Autodesk Inventor part; units mm, degrees
ref_plane "YZ Plane" through (0, 0, 0) normal (1, 0, 0) x (0, 1, 0)
ref_plane "XZ Plane" through (0, 0, 0) normal (0, 1, 0) x (-1, 0, 0)
ref_plane "XY Plane" through (0, 0, 0) normal (0, 0, 1) x (1, 0, 0)
sketch "Sketch1" plane through (0, 0, 0) normal (0, 1, 0) x (-1, 0, 0)
  circle A0 centre (0, 35) radius 7.5
  circle A1 centre (0, -35) radius 7.5
  circle A2 centre (0, 0) radius 6
  dimension "d0" = 15
  dimension "d1" = 35
  dimension "d2" = 15
  dimension "d3" = 35
  dimension "d4" = 12
sketch "Sketch2" plane through (0, 0, 0) normal (0, 1, 0) x (-1, 0, 0)
  line L0 (12, 40) -> (12, -40)
  line L1 (12, -40) -> (5, -55)
  line L2 (12, 40) -> (5, 55)
  line L3 (0, 53.0774) -> (0, -54.9051) construction
  line L4 (-12, 40) -> (-12, -40)
  line L5 (-12, -40) -> (-5, -55)
  line L6 (-12, 40) -> (-5, 55)
  arc A0 (5, 55) -> (-5, 55) centre (0, 52.6667) ccw
  arc A1 (-5, -55) -> (5, -55) centre (0, -52.6667) ccw
  point P0 (0, 0)
  dimension "d5" = 12
  dimension "d6" = 40
  dimension "d7" = 40
  dimension "d8" = 15
  dimension "d9" = 7
  dimension "d10" = 15
  dimension "d11" = 7
extrude "Extrusion1" add sketch "Sketch2" along normal blind 15
extrude "Extrusion2" cut sketch "Sketch1" along normal blind 10
sketch "Sketch3" plane through (0, 0, 0) normal (0, -1, 0) x (1, 0, 0)
  point P0 (0, 0)
  point P1 (0, -50)
  point P2 (0, 50)
  dimension "d16" = 50
  dimension "d17" = 50
hole "Hole1" at (0, 0, -50) at (0, 0, 50) direction (0, 1, 0) diameter 4 end through all counterbore diameter 5 counterbore depth 2
properties part number "Rahmen_Y_Halterung_v1"
Here's how the part is built. I have some questions about the finished solid (model axes, mm). A direction names the side the tool comes from. Give positions to 0.01 mm unless a question says otherwise; leave off trailing zeros. Loops run counter-clockwise (first coordinate to the right, second up) from the corner with the lowest first, then second, coordinate; pieces in that order, holes last. Notation, with made-up numbers: (25, -19.75) -> (51, -19.75) arc R10 cw to (51, -6.75) -> close; hole circle Ø6 at (-22, -30). An arc over 180 degrees is marked (long way). Use one line per item in the form item = value. Start each with the question number.
1) Imagine slicing it at B-B (z = -50). Please give me the cut outline in (x, y), then the cut area to 3 significant figures.
2) Which directions (+Z, -Z, +X, -X, +Y, -Y) give clear straight access to the entire face, cutting with the end or side of a thin tool? Please do faces 4 (the face through (-2, 2, 51)), 5 (the face through (12, 7, 1)).
3) Please list where these lines run through material, in increasing order: line 1 along Z through (x, y) = (1, 1.5); line 2 along Z through (x, y) = (2.25, 8.5).
4) Imagine slicing it at A-A (x = 0). Count the separate pieces of the cut face and the enclosed holes in it, then the cut area to 3 significant figures.
5) Imagine slicing it at D-D (z = 35). Please give me the cut outline in (x, y).
6) Thinking about a two-plate mould opening in X: for faces 1 (the face through (8.549, 7.395, -47.395)), 2 (the face through (0.766, 8.591, -51.847)), 3 (the face through (-8.549, 7.395, 47.395)), which applies, +X half, -X half, draft (parallel to the pull), parting line (faces both ways), or undercut?
7) Imagine slicing it at C-C (y = 3). Please give me the cut outline in (x, z).
8) For P1, Ø6, axis at x = 6, y = 4, coming from the -Z side; P2, Ø7.5, axis at x = 1.5, z = -37, coming from the -Y side; P3, Ø1.5, axis at x = 1, z = -49, coming from the -Y side, each with a flat end and sliding along its axis, tell me the tip position at first contact or that it passes through.
Check values:
q1.outline = (-7.33, 0) -> (-2.5, 0) -> (-2.5, 2) -> (-2, 2) -> (-2, 15) -> (-7.33, 15) -> close; (2, 2) -> (2.5, 2) -> (2.5, 0) -> (7.33, 0) -> (7.33, 15) -> (2, 15) -> close
q1.area = 158 mm^2
q2.face_4 = -Y
q2.face_5 = +Z, -Z, +X, +Y, -Y
q3.line_1 = -58.09 to -52.29, -47.71 to -42.43, -27.57 to -5.92, 5.92 to 27.57, 42.43 to 47.71, 52.29 to 58.09
q3.line_2 = -57.7 to -42.15, -27.85 to -5.56, 5.56 to 27.85, 42.15 to 57.7
q4.separate_pieces = 3
q4.enclosed_holes = 0
q4.area = 1,200 mm^2
q5.outline = (-12, 0) -> (-7.5, 0) -> (-7.5, 10) -> (7.5, 10) -> (7.5, 0) -> (12, 0) -> (12, 15) -> (-12, 15) -> close
q6.face_1 = +X half
q6.face_2 = undercut
q6.face_3 = -X half
q7.outline = (-12, -40) -> (-5, -55) arc R5.52 ccw to (5, -55) -> (12, -40) -> (12, 40) -> (5, 55) arc R5.52 ccw to (-5, 55) -> (-12, 40) -> close; hole circle Ø15 at (0, -35); hole circle Ø15 at (0, 35); hole circle Ø12 at (0, 0); hole circle Ø4 at (0, -50); hole circle Ø4 at (0, 50)
q8.P1 = -57.3
q8.P2 = 10
q8.P3 = 2
